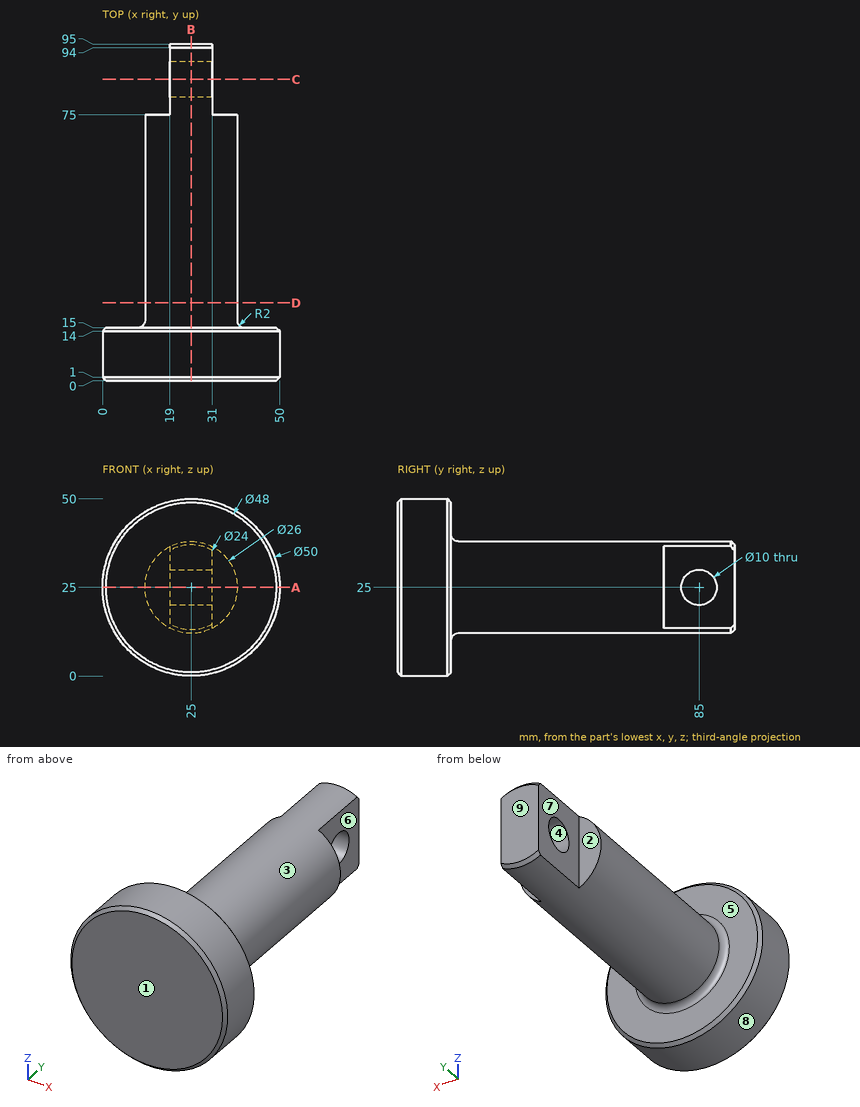
Here's the drawing with two shaded views (mm, measured from the low corner). I have some questions. A direction names the side the tool comes from. Coordinates: 2 decimals unless noted, no trailing zeros. Loops run counter-clockwise (first coordinate to the right, second up) from the corner with the lowest first, then second, coordinate; pieces in that order, holes last.
Item 1: Suppose I cut it at C-C (y = 85). Please give me the cut outline in (x, z).
Answers below:
outline: (19, 13.47) arc R13 ccw to (31, 13.47) - (31, 20) - (19, 20) - close; (19, 30) - (31, 30) - (31, 36.53) arc R13 ccw to (19, 36.53) - close
Item 2: I'm going to push flat-ended pins straight in: pin 1 (2 mm diameter, centred on x = 36, z = 23, fed in from +Y); pin 2 (5 mm diameter, centred on y = 38.5, z = 31.5, fed in from +X); pin 3 (12 mm diameter, centred on x = 37, y = 40, fed in from +Z); pin 4 (8 mm diameter, centred on y = 85, z = 25, fed in from -X). Where does each tip first touch, or does it pass through?
Answers below:
pin 1: stops at y = 75
pin 2: stops at x = 37.37
pin 3: stops at z = 36.53
pin 4: passes through
Item 3: Suppose I cut it at A-A (z = 25). Please give me the cut outline in (x, y), then the cut area to 3 significant figures.
Answers below:
outline: (0, 1) - (1, 0) - (49, 0) - (50, 1) - (50, 14) - (49, 15) - (40, 15) arc R2 cw to (38, 17) - (38, 75) - (31, 75) - (31, 80) - (19, 80) - (19, 75) - (12, 75) - (12, 17) arc R2 cw to (10, 15) - (1, 15) - (0, 14) - close; (19, 90) - (31, 90) - (31, 95) - (19, 95) - close
area: 2,430 mm2
Item 4: Suppose I cut it at D-D (y = 22). Please give me the cut outline in (x, z).
Answers below:
outline: circle Ø26 at (25, 25)
Item 5: If we mould it in two halves opening along Y, with no side actions, what happens to the marked faces 1, 2, 3 and 4? For each: released by +Y, released by -Y, zero draft, split by the parting line, or undercut.
Answers below:
face 1: released by -Y
face 2: released by +Y
face 3: zero draft
face 4: undercut
Item 6: Suppose I cut it at B-B (x = 25). Please give me the cut outline in (y, z).
Answers below:
outline: (0, 1) - (1, 0) - (14, 0) - (15, 1) - (15, 10) arc R2 cw to (17, 12) - (94, 12) - (95, 13) - (95, 37) - (94, 38) - (17, 38) arc R2 cw to (15, 40) - (15, 49) - (14, 50) - (1, 50) - (0, 49) - close; hole circle Ø10 at (85, 25)
Item 7: Which directions (+Z, -Z, +X, -X, +Y, -Y) give clear straight access to the entire face, cutting with the end or side of a thin tool? Please do the marked faces 5, 6, 7, 8 and 9.
Answers below:
face 5: +Y
face 6: +Z, -Z, +X, +Y
face 7: +Z, -Z, -X, +Y
face 8: +Y, -Y
face 9: +Z, -Z, +X, -X, +Y
Item 8: Please list where these lines run through material, in increasing order: L1, parallel to Y at x = 27, z = 25; L2, parallel to Y at x = 35, z = 26; L3, parallel to Y at x = 5, z = 21.
Answers below:
L1: y = 0 to 80, 90 to 95
L2: y = 0 to 75
L3: y = 0 to 15
